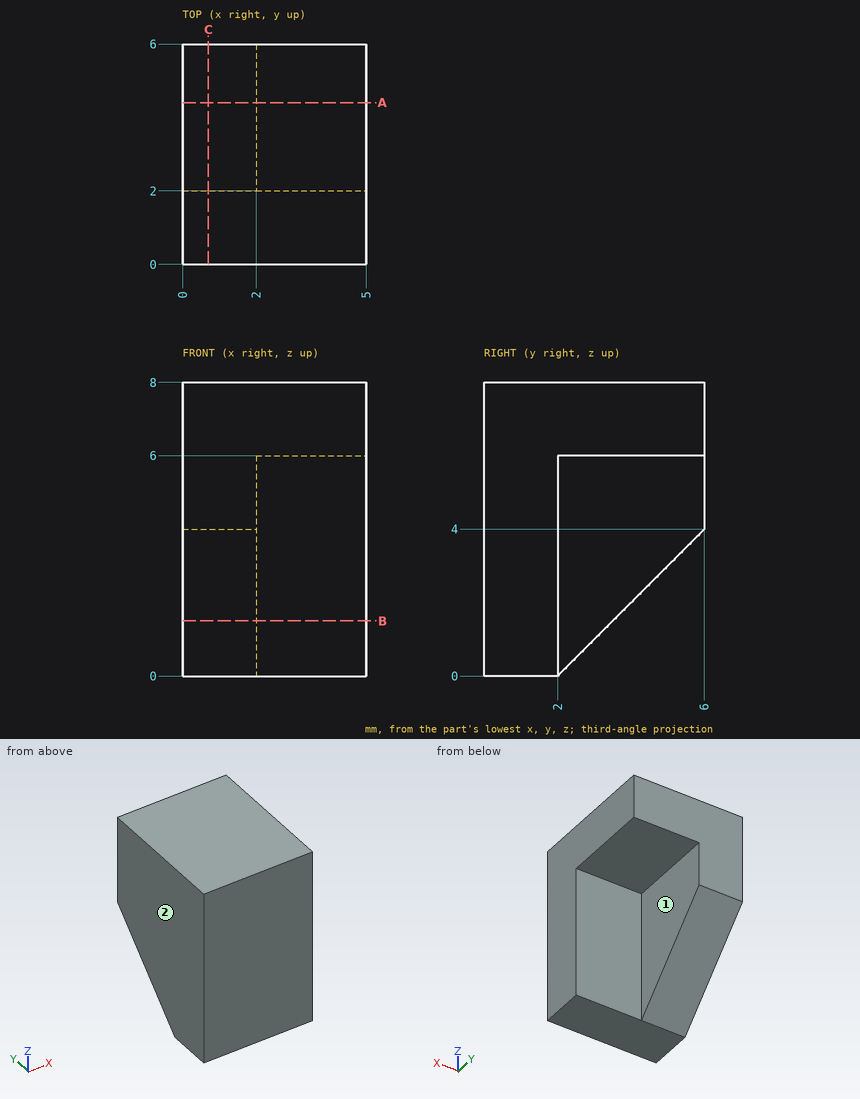
Could you check a few things on this drawing? It's one solid part, dimensions in mm from its lowest x, y, z. A direction names the side the tool comes from. Round coordinates to 2 decimals unless told otherwise and drop trailing zeros. Order: outer loops, then holes, each group sorted by start corner. A loop starts at its lowest first (then second) coordinate and runs counter-clockwise, first axis right, second up. Notation, with made-up numbers: M 51.5,39 L 58.5,39 A19 cw 58.5,76 Z; hole C 58.25,-15.5 d4. An arc over 180 degrees is marked long. Use a Markdown table: item, result.
1) If I drill on line 1 along X through (y, z) = (4.85, 4.25); line 2 along Z through (x, y) = (4.3, 2.2), over which ranges is the centre line in solid material (lowest first)?
Geometry says:
| item | result |
|---|---|
| line 1 | x = 0 to 2 |
| line 2 | z = 6 to 8 |
2) Imagine slicing it at B-B (z = 1.5). List the corners of the cut face in (x, y) for me, then the cut area to 3 significant figures.
Geometry says:
| item | result |
|---|---|
| outline | M 0,0 L 5,0 L 5,2 L 2,2 L 2,3.5 L 0,3.5 Z |
| area | 13.0 mm² |
3) Imagine slicing it at A-A (y = 4.4). List the corners of the cut face in (x, z) for me, then the cut area to 3 significant figures.
Geometry says:
| item | result |
|---|---|
| outline | M 0,2.4 L 2,2.4 L 2,6 L 5,6 L 5,8 L 0,8 Z |
| area | 17.2 mm² |
4) Imagine slicing it at C-C (x = 0.7). List the corners of the cut face in (y, z) for me.
Geometry says:
| item | result |
|---|---|
| outline | M 0,0 L 2,0 L 6,4 L 6,8 L 0,8 Z |
5) On a 3-axis mill with a long thin cutter (end or side, diameter ignored), from which of +Z, -Z, +X, -X, +Y, -Y can I reach the whole of each face in a straight line? I mean the marked faces 1 and 2. Say none if no direction works.
Geometry says:
| item | result |
|---|---|
| face 1 | -Z, +X, +Y |
| face 2 | +Z, -Z, -X, +Y, -Y |
6) I'm going to push flat-ended pins straight in: P1, Ø1.5, axis at x = 4, z = 3.5, coming from the +Y side; P2, Ø2.5, axis at x = 3.5, y = 4, coming from the -Z side; P3, Ø1.2, axis at y = 3, z = 2.5, coming from the +X side. Where does each tip first touch, or does it pass through?
Geometry says:
| item | result |
|---|---|
| P1 | stops at y = 2 |
| P2 | stops at z = 6 |
| P3 | stops at x = 2 |
